For this review, take the finished solid that the model builds, in its own axes (mm). Give positions to 0.01 mm unless a question says otherwise; leave off trailing zeros. Loops run counter-clockwise (first coordinate to the right, second up) from the corner with the lowest first, then second, coordinate; pieces in that order, holes last. Notation, with made-up numbers: (-4, 32) -> (31, 32) arc R19 cw to (31, 44) -> close; hole circle Ø7 at (32.5, -24). An arc over 180 degrees is marked (long way). One line per question, with ' | ' between items. Start each with the question number.
(1) Consider section C-C (z = 90.5). Write out the cut boundary in (x, y).
(2) Consider section A-A (y = 0.45). Write out the cut boundary in (x, z), and give its area (3 significant figures).
(3) Consider section B-B (x = -3.5). Write out the cut boundary in (y, z).
(4) Wall thickness on probe 1 along X at (y, z) = (0.2, 102.5); probe 2 along Z at (x, y) = (27.5, 0.6); probe 3 along Z at (x, y) = (-2, 0.4): over which ranges is each line inside the solid? List them lowest first.
(5) Insertion check: P1, Ø0.8, axis at y = 1, z = 76.5, coming from the +X side; P2, Ø3, axis at x = -7, z = 81, coming from the -Y side. Each pin has a flat end and moves straight along its axis. Give the tip position at first contact, or say it passes through.
from build123d import *

# Parameters (mm, degrees)
BOSS_EXTRUDE1_DEPTH = 1.5
FILLET1_R           = 2


with BuildPart() as part:
    # Sketch1 → Boss-Extrude1 (new body)
    with BuildSketch(Plane(origin=(0, 0, 0), x_dir=(1, 0, 0), z_dir=(0, 1, 0))):
        Polygon((0, 0), (35, -35), (15, -35), (15, -110), (-15, -110), (-15, -35), (-35, -35), align=None)
    extrude(amount=BOSS_EXTRUDE1_DEPTH)

    # Fillet1
    fillet1_edges = [part.edges().sort_by_distance(p)[0] for p in [
        (0, 0.75, 0),
        (35, 0.75, 35),
        (15, 0.75, 35),
        (15, 0.75, 110),
        (-15, 0.75, 110),
        (-15, 0.75, 35),
        (-35, 0.75, 35),
    ]]
    fillet(fillet1_edges, radius=FILLET1_R)


solid = part.part
A:
1) outline: (-15, 0) -> (15, 0) -> (15, 1.5) -> (-15, 1.5) -> close
2) outline: (-31.59, 31.59) -> (-1.41, 1.41) arc R2 ccw to (1.41, 1.41) -> (31.59, 31.59) arc R2 ccw to (30.17, 35) -> (17, 35) arc R2 cw to (15, 37) -> (15, 108) arc R2 ccw to (13, 110) -> (-13, 110) arc R2 ccw to (-15, 108) -> (-15, 37) arc R2 cw to (-17, 35) -> (-30.17, 35) arc R2 ccw to start | area: 3,460 mm^2
3) outline: (0, 3.5) -> (1.5, 3.5) -> (1.5, 110) -> (0, 110) -> close
4) probe 1: x = -15 to 15 | probe 2: z = 27.5 to 35 | probe 3: z = 2 to 110
5) P1: stops at x = 15 | P2: stops at y = 0
